from build123d import *

# Parameters (mm, degrees)
F0_W     = 45
F0_H     = 45
F1_DEPTH = 100
F2_W     = 25
F2_H     = 25
F3_DEPTH = 63
F4_W     = 5.842124
F4_H     = 25.543576
F5_DEPTH = 10


with BuildPart() as f1:
    # F0 (on Top) → F1 (new body)
    with BuildSketch(Plane.XY):
        Rectangle(F0_W, F0_H)
    extrude(amount=F1_DEPTH)

    # F2 (on face) → F3 (cut)
    with BuildSketch(Plane.XY.offset(100)):
        Rectangle(F2_W, F2_H)
    extrude(amount=-F3_DEPTH, mode=Mode.SUBTRACT)

    # F4 (on face) → F5 (cut)
    with BuildSketch(Plane.XZ.offset(22.5)):
        with Locations((-0.454231, 87.228212)):
            Rectangle(F4_W, F4_H)
    extrude(amount=-F5_DEPTH, mode=Mode.SUBTRACT)


solid = f1.part
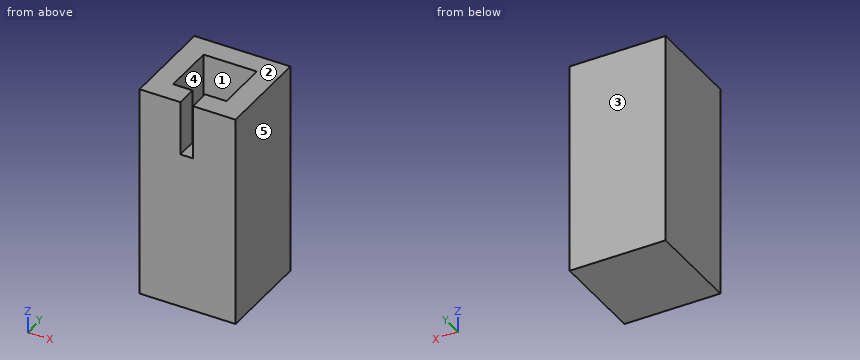
The model under review builds one solid part; all positions refer to its coordinate system, in mm. Face numbers are marked on the shaded views. A direction names the side the tool comes from. Give positions to 0.01 mm unless a question says otherwise; leave off trailing zeros. Loops run counter-clockwise (first coordinate to the right, second up) from the corner with the lowest first, then second, coordinate; pieces in that order, holes last. Notation, with made-up numbers: (-39.75, 70.5) -> (11.25, 70.5) arc R29 cw to (11.25, 107.5) -> close; hole circle Ø8 at (-10, 64). An arc over 180 degrees is marked (long way). Answer as a JSON object with one key per item and string values. Group by question number.
Q1. Take a section at A-A (z = 54). Write out the cut boundary in (x, y), plus the area to 3 significant figures.
Q2. Wall thickness on line 1 along X through (y, z) = (10.5, 86.5); line 2 along Z through (x, y) = (-6, 10): over which ranges is each line inside the solid? List them lowest first.
Q3. Take a section at D-D (z = 88.5). Write out the cut boundary in (x, y).
Q4. Insertion check: pin 1 (12.5 mm diameter, centred on x = -3, y = -5, fed in from +Z). The pin has a flat end and moves straight along its axis. Give the tip position at first contact, or say it passes through.
Q5. Take a section at B-B (x = -6). Write out the cut boundary in (y, z).
Q6. Draft analysis for pull direction X (two halves, no side actions). For the marked faces 3, 4 and 5, state which applies: pulls with the +X half, pulls with the -X half, needs draft (parallel to the pull), parting line crosses it, or undercut.
Q7. Tool access review of the marked faces 1 and 2: name each direction out of +Z, -Z, +X, -X, +Y, -Y from which nothing blocks a thin tool from reaching the whole face with its end or side.
Answer below:
{
 "1": {"outline": "(-22.5, -22.5) -> (22.5, -22.5) -> (22.5, 22.5) -> (-22.5, 22.5) -> close; hole (-12.5, -12.5) -> (12.5, -12.5) -> (12.5, 12.5) -> (-12.5, 12.5) -> close", "area": "1,400 mm2"},
 "2": {"line 1": "x = -22.5 to -12.5, 12.5 to 22.5", "line 2": "z = 0 to 37"},
 "3": {"outline": "(-22.5, -22.5) -> (-3.38, -22.5) -> (-3.38, -12.5) -> (-12.5, -12.5) -> (-12.5, 12.5) -> (12.5, 12.5) -> (12.5, -12.5) -> (2.47, -12.5) -> (2.47, -22.5) -> (22.5, -22.5) -> (22.5, 22.5) -> (-22.5, 22.5) -> close"},
 "4": {"pin 1": "stops at z = 37"},
 "5": {"outline": "(-22.5, 0) -> (22.5, 0) -> (22.5, 100) -> (12.5, 100) -> (12.5, 37) -> (-12.5, 37) -> (-12.5, 100) -> (-22.5, 100) -> close"},
 "6": {"face 3": "needs draft", "face 4": "undercut", "face 5": "pulls with the +X half"},
 "7": {"face 1": "+Z", "face 2": "+Z, +X, -X, +Y, -Y"}
}
